Part model, mm, in its own coordinate system. Round coordinates to 2 decimals unless told otherwise and drop trailing zeros. Loops run counter-clockwise (first coordinate to the right, second up) from the corner with the lowest first, then second, coordinate; pieces in that order, holes last.
from build123d import *

# Parameters (mm, degrees)
F0_W     = 124
F0_H     = 124
F0_W_2   = 42
F0_H_2   = 15.5
F1_DEPTH = 2


with BuildPart() as f1:
    # F0 (on Top) → F1 (new body, symmetric)
    with BuildSketch(Plane.XY):
        Rectangle(F0_W, F0_H)
        with Locations((-31, -46.5)):
            Rectangle(F0_W_2, F0_H_2, mode=Mode.SUBTRACT)
        with Locations((-21, -23.25)):
            Rectangle(F0_W_2, F0_H_2, mode=Mode.SUBTRACT)
        with Locations((21, -46.5)):
            Rectangle(F0_W_2, F0_H_2, mode=Mode.SUBTRACT)
        with Locations((31, -23.25)):
            Rectangle(F0_W_2, F0_H_2, mode=Mode.SUBTRACT)
        with Locations((-31, 0)):
            Rectangle(F0_W_2, F0_H_2, mode=Mode.SUBTRACT)
        with Locations((-21, 23.25)):
            Rectangle(F0_W_2, F0_H_2, mode=Mode.SUBTRACT)
        with Locations((-31, 46.5)):
            Rectangle(F0_W_2, F0_H_2, mode=Mode.SUBTRACT)
        with Locations((21, 0)):
            Rectangle(F0_W_2, F0_H_2, mode=Mode.SUBTRACT)
        with Locations((31, 23.25)):
            Rectangle(F0_W_2, F0_H_2, mode=Mode.SUBTRACT)
        with Locations((21, 46.5)):
            Rectangle(F0_W_2, F0_H_2, mode=Mode.SUBTRACT)
    extrude(amount=F1_DEPTH, both=True)


solid = f1.part
1) Wall check: line 1 along X through (y, z) = (28, -0.95); line 2 along Y through (x, z) = (-34, 1.6); line 3 along X through (y, z) = (42, 1.6). Give the ranges that are in metal, low to high.
Values:
line 1: x = -62 to -42, 0 to 10, 52 to 62
line 2: y = -62 to -54.25, -38.75 to -31, -15.5 to -7.75, 7.75 to 15.5, 31 to 38.75, 54.25 to 62
line 3: x = -62 to -52, -10 to 0, 42 to 62
2) Slice it at D-D, the plane z = 0.15. Give the number of separate pieces and of enclosed holes in the cut face, then the cut area to 3 significant figures.
Values:
separate pieces: 1
enclosed holes: 10
area: 8,870 mm2
3) Slice it at C-C, the plane x = -6.5. Give the cut face in (y, z), then the cut area to 3 significant figures.
Values:
outline: (-62, -2) - (-31, -2) - (-31, 2) - (-62, 2) - close; (-15.5, -2) - (15.5, -2) - (15.5, 2) - (-15.5, 2) - close; (31, -2) - (62, -2) - (62, 2) - (31, 2) - close
area: 372 mm2
4) Slice it at A-A, the plane x = 21.5. Give the cut face in (y, z), then the cut area to 3 significant figures.
Values:
outline: (-62, -2) - (-54.25, -2) - (-54.25, 2) - (-62, 2) - close; (-38.75, -2) - (-31, -2) - (-31, 2) - (-38.75, 2) - close; (-15.5, -2) - (-7.75, -2) - (-7.75, 2) - (-15.5, 2) - close; (7.75, -2) - (15.5, -2) - (15.5, 2) - (7.75, 2) - close; (31, -2) - (38.75, -2) - (38.75, 2) - (31, 2) - close; (54.25, -2) - (62, -2) - (62, 2) - (54.25, 2) - close
area: 186 mm2
5) Slice it at B-B, the plane y = 25. Give the cut face in (x, z), then the cut area to 3 significant figures.
Values:
outline: (-62, -2) - (-42, -2) - (-42, 2) - (-62, 2) - close; (0, -2) - (10, -2) - (10, 2) - (0, 2) - close; (52, -2) - (62, -2) - (62, 2) - (52, 2) - close
area: 160 mm2
6) Drop a flat-ended pin along its axis: pin 1 Ø12 at (x, y) = (38.5, -23) entering from -Z. Give the stop position or say it passes through.
Values:
pin 1: passes through
